from build123d import *

# Parameters (mm, degrees)
ESQUISSE1_W                                   = 160
ESQUISSE1_H                                   = 120
BOSS_EXTRU_1_DEPTH                            = 8
ESQUISSE2_W                                   = 32
ESQUISSE2_H                                   = 32
ENL_V_MAT_EXTRU_1_DEPTH                       = 5.7
ENL_V_MAT_EXTRU_2_DEPTH                       = 3
TROU_POUR_TARAUDAGE_POUR_TROU_TARAUD_M5_D     = 4.2
TROU_POUR_TARAUDAGE_POUR_TROU_TARAUD_M5_DEPTH = 8
TROU_POUR_TARAUDAGE_POUR_TROU_TARAUD_M5_TIP   = 1.2618073
CONG_1_R                                      = 1
ESQUISSE7_R                                   = 2.845
ENL_V_MAT_EXTRU_3_DEPTH                       = 6


with BuildPart() as part:
    # Esquisse1 → Boss.-Extru.1 (new body)
    with BuildSketch(Plane.XY):
        with Locations((-7.227655867, -5.967741935)):
            Rectangle(ESQUISSE1_W, ESQUISSE1_H)
    extrude(amount=BOSS_EXTRU_1_DEPTH)

    # Esquisse2 → Enlèv. mat.-Extru.1 (cut)
    with BuildSketch(Plane.XY.offset(8)):
        with Locations((-24.227655867, 15.032258065)):
            Rectangle(ESQUISSE2_W, ESQUISSE2_H)
        with Locations((-58.227655867, 15.032258065)):
            Rectangle(ESQUISSE2_W, ESQUISSE2_H)
        with Locations((9.772344133, 15.032258065)):
            Rectangle(ESQUISSE2_W, ESQUISSE2_H)
        with Locations((43.772344133, 15.032258065)):
            Rectangle(ESQUISSE2_W, ESQUISSE2_H)
        with Locations((-24.227655867, -18.967741935)):
            Rectangle(ESQUISSE2_W, ESQUISSE2_H)
        with Locations((9.772344133, -18.967741935)):
            Rectangle(ESQUISSE2_W, ESQUISSE2_H)
        with Locations((43.772344133, -18.967741935)):
            Rectangle(ESQUISSE2_W, ESQUISSE2_H)
        with Locations((-58.227655867, -18.967741935)):
            Rectangle(ESQUISSE2_W, ESQUISSE2_H)
    extrude(amount=-ENL_V_MAT_EXTRU_1_DEPTH, mode=Mode.SUBTRACT)

    # Esquisse3 → Enlèv. mat.-Extru.2 (cut)
    with BuildSketch(Plane.XY.offset(8)):
        with BuildLine():
            Line((-68.227655867, 49.032258065), (53.772344133, 49.032258065))
            ThreePointArc((53.772344133, 49.032258065), (63.67183907, 44.931753001), (67.772344133, 35.032258065))
            Line((67.772344133, 35.032258065), (67.772344133, -47.967741935))
            ThreePointArc((67.772344133, -47.967741935), (63.67183907, -57.867236872), (53.772344133, -61.967741935))
            Line((53.772344133, -61.967741935), (-68.227655867, -61.967741935))
            ThreePointArc((-68.227655867, -61.967741935), (-78.127150803, -57.867236872), (-82.227655867, -47.967741935))
            Line((-82.227655867, -47.967741935), (-82.227655867, 35.032258065))
            ThreePointArc((-82.227655867, 35.032258065), (-78.127150803, 44.931753001), (-68.227655867, 49.032258065))
        make_face()
        with BuildLine():
            Line((-79.227655867, 35.032258065), (-79.227655867, -47.967741935))
            ThreePointArc((-79.227655867, -47.967741935), (-76.00583046, -55.745916529), (-68.227655867, -58.967741935))
            Line((-68.227655867, -58.967741935), (53.772344133, -58.967741935))
            ThreePointArc((53.772344133, -58.967741935), (61.550518726, -55.745916529), (64.772344133, -47.967741935))
            Line((64.772344133, -47.967741935), (64.772344133, 35.032258065))
            ThreePointArc((64.772344133, 35.032258065), (61.550518726, 42.810432658), (53.772344133, 46.032258065))
            Line((53.772344133, 46.032258065), (-68.227655867, 46.032258065))
            ThreePointArc((-68.227655867, 46.032258065), (-76.00583046, 42.810432658), (-79.227655867, 35.032258065))
        make_face(mode=Mode.SUBTRACT)
    extrude(amount=-ENL_V_MAT_EXTRU_2_DEPTH, mode=Mode.SUBTRACT)

    # Trou pour taraudage pour trou taraudé M51
    with Locations(Plane.XY.offset(8)):
        with Locations((-81.227655867, -59.967741935), (-81.227655867, 48.032258065), (66.772344133, 48.032258065), (66.772344133, -59.967741935)):
            Hole(TROU_POUR_TARAUDAGE_POUR_TROU_TARAUD_M5_D / 2, depth=TROU_POUR_TARAUDAGE_POUR_TROU_TARAUD_M5_DEPTH)
            with Locations((0, 0, -(TROU_POUR_TARAUDAGE_POUR_TROU_TARAUD_M5_DEPTH + TROU_POUR_TARAUDAGE_POUR_TROU_TARAUD_M5_TIP / 2))):  # 118° drill point
                Cone(0, TROU_POUR_TARAUDAGE_POUR_TROU_TARAUD_M5_D / 2, TROU_POUR_TARAUDAGE_POUR_TROU_TARAUD_M5_TIP, mode=Mode.SUBTRACT)

    # Congé1
    cong_1_edges = [part.edges().sort_by_distance(p)[0] for p in [
        (-74.227655867, -0.967741935, 5.15),
        (-74.227655867, 31.032258065, 5.15),
        (-42.227655867, 31.032258065, 5.15),
        (-42.227655867, -0.967741935, 5.15),
        (-40.227655867, -0.967741935, 5.15),
        (-40.227655867, 31.032258065, 5.15),
        (-8.227655867, 31.032258065, 5.15),
        (-8.227655867, -0.967741935, 5.15),
        (-6.227655867, -0.967741935, 5.15),
        (-6.227655867, 31.032258065, 5.15),
        (25.772344133, 31.032258065, 5.15),
        (25.772344133, -0.967741935, 5.15),
        (27.772344133, -0.967741935, 5.15),
        (27.772344133, 31.032258065, 5.15),
        (59.772344133, 31.032258065, 5.15),
        (59.772344133, -0.967741935, 5.15),
        (-74.227655867, -34.967741935, 5.15),
        (-74.227655867, -2.967741935, 5.15),
        (-42.227655867, -2.967741935, 5.15),
        (-42.227655867, -34.967741935, 5.15),
        (27.772344133, -34.967741935, 5.15),
        (27.772344133, -2.967741935, 5.15),
        (59.772344133, -2.967741935, 5.15),
        (59.772344133, -34.967741935, 5.15),
        (-6.227655867, -34.967741935, 5.15),
        (-6.227655867, -2.967741935, 5.15),
        (25.772344133, -2.967741935, 5.15),
        (25.772344133, -34.967741935, 5.15),
        (-40.227655867, -34.967741935, 5.15),
        (-40.227655867, -2.967741935, 5.15),
        (-8.227655867, -2.967741935, 5.15),
        (-8.227655867, -34.967741935, 5.15),
    ]]
    fillet(cong_1_edges, radius=CONG_1_R)

    # Esquisse7 → Enlèv. mat.-Extru.3 (cut)
    with BuildSketch(Plane.XY.offset(8)):
        with Locations((-72.727655867, 35.832258065)):
            Circle(ESQUISSE7_R)
        with Locations((-72.727655867, -38.967741935)):
            Circle(ESQUISSE7_R)
        with Locations((58.272344133, -38.967741935)):
            Circle(ESQUISSE7_R)
        with Locations((58.272344133, 35.832258065)):
            Circle(ESQUISSE7_R)
    extrude(amount=-ENL_V_MAT_EXTRU_3_DEPTH, mode=Mode.SUBTRACT)


solid = part.part
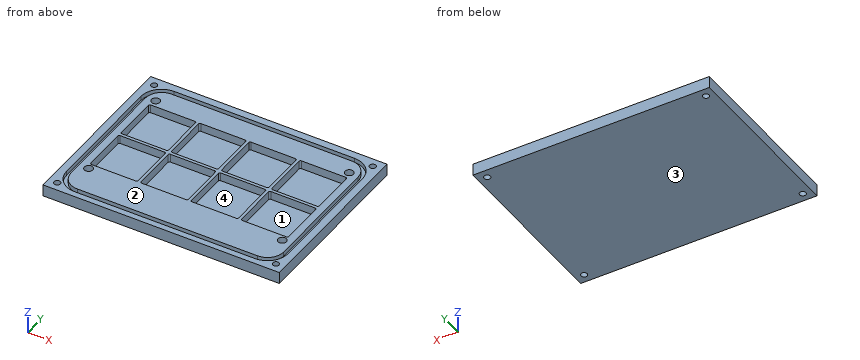
Read the model definition and answer for the solid it produces. Units are mm, in the model's axes. Face numbers are marked on the shaded views. A direction names the side the tool comes from. Round coordinates to 2 decimals unless told otherwise and drop trailing zeros. Write each loop counter-clockwise with the first axis right and the second up, starting at its lowest first coordinate (ties: lowest second). Pieces come first, ordered by that corner, then holes. Notation, with made-up numbers: M -30.5,70.25 L 23.5,70.25 A23 ccw 23.5,88.25 Z; hole C 11,52 d6. An arc over 180 degrees is marked long. Use a Markdown table: item, result.
1) For a pull along X with two mould halves and no side action, classify the marked faces 3 and 4 as pulls with the +X half, pulls with the -X half, needs draft (parallel to the pull), parting line crosses it, or undercut.
Answers follow:
| item | result |
|---|---|
| face 3 | needs draft |
| face 4 | undercut |
2) A tool of negligible diameter and unlimited length cuts with its end or side. For the marked faces 1 and 2, from which of +Z, -Z, +X, -X, +Y, -Y can it reach the whole face along a straight path? Write none if from no direction.
Answers follow:
| item | result |
|---|---|
| face 1 | +Z |
| face 2 | +Z, +X, -X, +Y, -Y |
3) The part is cut by section C-C (z = 3.75). Give the number of separate pieces and of enclosed holes in the cut face, plus the area to 3 significant figures.
Answers follow:
| item | result |
|---|---|
| separate pieces | 1 |
| enclosed holes | 16 |
| area | 10,900 mm2 |
4) The part is cut by section D-D (y = 43.5). Write down the section's boundary in (x, z).
Answers follow:
| item | result |
|---|---|
| outline | M -87.23,0 L 72.77,0 L 72.77,8 L 64.92,8 L 64.92,5 L 60.79,5 L 60.79,8 L -75.25,8 L -75.25,5 L -79.38,5 L -79.38,8 L -87.23,8 Z |
5) Straight lines are drawn through the part: line 1 along Y through (x, z) = (-46, 6.25); line 2 along Y through (x, z) = (49, 3.5); line 3 along X through (y, z) = (31.5, 7.25). For each, find the intervals that lie inside material, in ascending order. Write a range as [from, to].
Answers follow:
| item | result |
|---|---|
| line 1 | y = [-65.97, -61.97], [-58.97, -34.97], [-2.97, -0.97], [31.03, 46.03], [49.03, 54.03] |
| line 2 | y = [-65.97, -34.97], [-2.97, -0.97], [31.03, 54.03] |
| line 3 | x = [-87.23, -82.23], [-79.23, 64.77], [67.77, 72.77] |
6) A flat-ended cylindrical pin translates along its axis: pin 1 (1.7 mm diameter, centred on x = 58.5, y = 35, fed in from +Z). Find the tip coordinate at first contact, or state that the pin passes through.
Answers follow:
| item | result |
|---|---|
| pin 1 | stops at z = 2 |
7) The part is cut by section B-B (y = -10). Write down the section's boundary in (x, z), plus the area to 3 significant figures.
Answers follow:
| item | result |
|---|---|
| outline | M -87.23,0 L 72.77,0 L 72.77,8 L 67.77,8 L 67.77,5 L 64.77,5 L 64.77,8 L 59.77,8 L 59.77,2.3 L 27.77,2.3 L 27.77,8 L 25.77,8 L 25.77,2.3 L -6.23,2.3 L -6.23,8 L -8.23,8 L -8.23,2.3 L -40.23,2.3 L -40.23,8 L -42.23,8 L -42.23,2.3 L -74.23,2.3 L -74.23,8 L -79.23,8 L -79.23,5 L -82.23,5 L -82.23,8 L -87.23,8 Z |
| area | 532 mm2 |
8) The part is cut by section A-A (x = 43). Write down the section's boundary in (y, z).
Answers follow:
| item | result |
|---|---|
| outline | M -65.97,0 L 54.03,0 L 54.03,8 L 49.03,8 L 49.03,5 L 46.03,5 L 46.03,8 L 31.03,8 L 31.03,2.3 L -0.97,2.3 L -0.97,8 L -2.97,8 L -2.97,2.3 L -34.97,2.3 L -34.97,8 L -58.97,8 L -58.97,5 L -61.97,5 L -61.97,8 L -65.97,8 Z |
